Work out the finished part from the listing and answer in its coordinate system (mm). A direction names the side the tool comes from. Coordinates: 2 decimals unless noted, no trailing zeros. Loops run counter-clockwise (first coordinate to the right, second up) from the corner with the lowest first, then second, coordinate; pieces in that order, holes last. Notation, with made-up numbers: (87.25, 33.5) -> (96.25, 33.5) arc R15 cw to (96.25, 47.5) -> close; hole circle Ø4 at (23, -4). An arc over 180 degrees is marked (long way). Use a Markdown table: item, result.
from build123d import *

# Parameters (mm, degrees)
SKETCH1_W           = 50
SKETCH1_H           = 20
BOSS_EXTRUDE1_DEPTH = 14
SKETCH2_W           = 50
SKETCH2_H           = 3
CUT_EXTRUDE1_DEPTH  = 14
SKETCH3_W           = 7
SKETCH3_H           = 8
CUT_EXTRUDE2_DEPTH  = 14
SKETCH4_W           = 38
SKETCH4_H           = 8
BOSS_EXTRUDE2_DEPTH = 4
FILLET2_R           = 2
SKETCH5_R           = 0.75
SKETCH5_R_2         = 0.775
CUT_EXTRUDE3_DEPTH  = 10


with BuildPart() as part:
    # Sketch1 → Boss-Extrude1 (new body)
    with BuildSketch(Plane(origin=(0, 0, 0), x_dir=(1, 0, 0), z_dir=(0, 1, 0))):
        with Locations((25, 10)):
            Rectangle(SKETCH1_W, SKETCH1_H)
    extrude(amount=BOSS_EXTRUDE1_DEPTH)

    # Sketch2 → Cut-Extrude1 (cut)
    with BuildSketch(Plane(origin=(0, 0, -20), x_dir=(-1, 0, 0), z_dir=(0, 0, -1))):
        with Locations((-25, 12.5)):
            Rectangle(SKETCH2_W, SKETCH2_H)
        with Locations((-25, 1.5)):
            Rectangle(SKETCH2_W, SKETCH2_H)
    extrude(amount=-CUT_EXTRUDE1_DEPTH, mode=Mode.SUBTRACT)

    # Sketch3 → Cut-Extrude2 (cut)
    with BuildSketch(Plane(origin=(0, 0, -20), x_dir=(-1, 0, 0), z_dir=(0, 0, -1))):
        with Locations((-3.5, 7)):
            Rectangle(SKETCH3_W, SKETCH3_H)
        with Locations((-46.5, 7)):
            Rectangle(SKETCH3_W, SKETCH3_H)
    extrude(amount=-CUT_EXTRUDE2_DEPTH, mode=Mode.SUBTRACT)

    # Sketch4 → Boss-Extrude2 (add)
    with BuildSketch(Plane.XY):
        with Locations((25, 6.990304204)):
            Rectangle(SKETCH4_W, SKETCH4_H)
    extrude(amount=BOSS_EXTRUDE2_DEPTH)

    # Fillet2
    fillet2_edges = [part.edges().sort_by_distance(p)[0] for p in [
        (44, 2.990304204, 2),
        (44, 10.990304204, 2),
        (6, 10.990304204, 2),
        (6, 2.990304204, 2),
    ]]
    fillet(fillet2_edges, radius=FILLET2_R)

    # Sketch5 → Cut-Extrude3 (cut)
    with BuildSketch(Plane.XY.offset(4)):
        with Locations((42.5, 9.355857952)):
            Circle(SKETCH5_R)
        with Locations((41, 4.690304204)):
            Circle(SKETCH5_R_2)
        with Locations((38, 4.690304204)):
            Circle(SKETCH5_R_2)
        with Locations((39.5, 9.355857952)):
            Circle(SKETCH5_R)
        with Locations((35, 4.690304204)):
            Circle(SKETCH5_R_2)
        with Locations((36.5, 9.355857952)):
            Circle(SKETCH5_R)
        with Locations((32, 4.690304204)):
            Circle(SKETCH5_R_2)
        with Locations((33.5, 9.355857952)):
            Circle(SKETCH5_R)
        with Locations((29, 4.690304204)):
            Circle(SKETCH5_R_2)
        with Locations((30.5, 9.355857952)):
            Circle(SKETCH5_R)
        with Locations((26, 4.690304204)):
            Circle(SKETCH5_R_2)
        with Locations((27.5, 9.355857952)):
            Circle(SKETCH5_R)
        with Locations((23, 4.690304204)):
            Circle(SKETCH5_R_2)
        with Locations((24.5, 9.355857952)):
            Circle(SKETCH5_R)
        with Locations((20, 4.690304204)):
            Circle(SKETCH5_R_2)
        with Locations((21.5, 9.355857952)):
            Circle(SKETCH5_R)
        with Locations((17, 4.690304204)):
            Circle(SKETCH5_R_2)
        with Locations((18.5, 9.355857952)):
            Circle(SKETCH5_R)
        with Locations((14, 4.690304204)):
            Circle(SKETCH5_R_2)
        with Locations((15.5, 9.355857952)):
            Circle(SKETCH5_R)
        with Locations((11, 4.690304204)):
            Circle(SKETCH5_R_2)
        with Locations((12.5, 9.355857952)):
            Circle(SKETCH5_R)
        with Locations((8, 4.690304204)):
            Circle(SKETCH5_R_2)
        with Locations((9.5, 9.355857952)):
            Circle(SKETCH5_R)
    extrude(amount=-CUT_EXTRUDE3_DEPTH, mode=Mode.SUBTRACT)


solid = part.part
Q1. Section C-C on z = 1 is taken. State how many separate pieces and enclosed holes the cut face has, and give its area (3 significant figures).
Solved:
| item | result |
|---|---|
| separate pieces | 1 |
| enclosed holes | 24 |
| area | 257 mm² |
Q2. Section D-D on z = -15.5 is taken. Determine the outline of the cut face in (x, y), and give its area (3 significant figures).
Solved:
| item | result |
|---|---|
| outline | (7, 3) -> (43, 3) -> (43, 11) -> (7, 11) -> close |
| area | 288 mm² |
Q3. Determine the mould class of faces 1 (the flat face through (33.5, 9.4, -6)), 2 (the flat face through (44, 7, 2)), 3 (the flat face through (39.5, 9.4, -6)), 4 (the flat face through (25, 7, 4)) for opening direction X: pulls with the +X half, pulls with the -X half, needs draft (parallel to the pull), parting line crosses it, or undercut.
Solved:
| item | result |
|---|---|
| face 1 | undercut |
| face 2 | pulls with the +X half |
| face 3 | undercut |
| face 4 | needs draft |
Q4. For faces 5 (the cylindrical face through (6.57, 10.39, 2.03)), 6 (the flat face through (25, 7, -20)), 7 (the cylindrical face through (23.74, 4.92, -0.93)), determine the directions among +Z, -Z, +X, -X, +Y, -Y from which every point of the face is accessible in a straight line to the end or side of a thin tool.
Solved:
| item | result |
|---|---|
| face 5 | +Z, -X, +Y |
| face 6 | -Z, +X, -X, +Y, -Y |
| face 7 | +Z |
Q5. Consider line 1 (Y direction, x = 26, z = 0.75); line 2 (Y direction, x = 33.5, z = -0.25); line 3 (Z direction, x = 44, y = 2.5). Determine where each line is inside the solid, lowest interval first. Write a range as [from, to].
Solved:
| item | result |
|---|---|
| line 1 | [2.99, 3.92], [5.47, 10.99] |
| line 2 | [0, 8.61], [10.11, 14] |
| line 3 | [-6, 0] |
Q6. Given pin 1 Ø0.9 at (x, y) = (20, 4.69) entering from +Z; pin 2 Ø12 at (x, z) = (21, -16.5) entering from +Y; pin 3 Ø3 at (x, z) = (27, 2) entering from -Y, each flat-ended and moving along its own axis, determine where each tip first touches the part or whether it passes through.
Solved:
| item | result |
|---|---|
| pin 1 | z = -6 |
| pin 2 | y = 11 |
| pin 3 | y = 2.99 |
Q7. Section B-B on y = 7.25 is taken. Determine the outline of the cut face in (x, z), and give its area (3 significant figures).
Solved:
| item | result |
|---|---|
| outline | (0, -6) -> (7, -6) -> (7, -20) -> (43, -20) -> (43, -6) -> (50, -6) -> (50, 0) -> (44, 0) -> (44, 4) -> (6, 4) -> (6, 0) -> (0, 0) -> close |
| area | 956 mm² |
Q8. Section A-A on x = 15.5 is taken. Determine the outline of the cut face in (y, z), and give its area (3 significant figures).
Solved:
| item | result |
|---|---|
| outline | (0, -6) -> (3, -6) -> (3, -20) -> (11, -20) -> (11, -6) -> (14, -6) -> (14, 0) -> (10.99, 0) -> (10.99, 4) -> (10.11, 4) -> (10.11, -6) -> (8.61, -6) -> (8.61, 4) -> (2.99, 4) -> (2.99, 0) -> (0, 0) -> close |
| area | 213 mm² |
